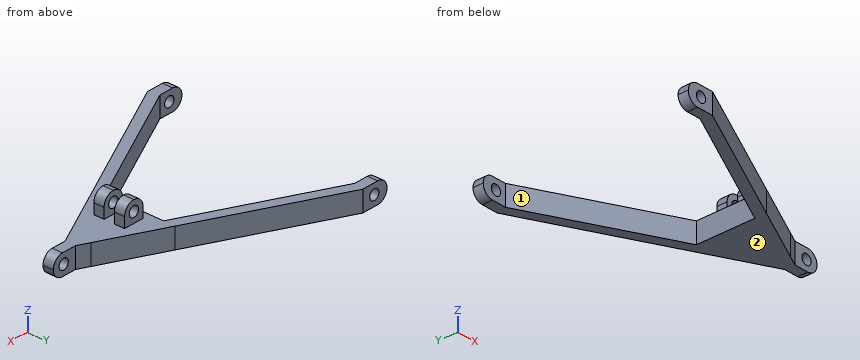
from build123d import *

# Parameters (mm, degrees)
EXTRUDE_THIN4_DEPTH = 20
SKETCH2_R           = 5
CUT_EXTRUDE1_DEPTH  = 235
BOSS_EXTRUDE1_DEPTH = 20
SKETCH4_W           = 20
SKETCH4_H           = 10
BOSS_EXTRUDE2_DEPTH = 20
SKETCH5_R           = 5
CUT_EXTRUDE2_DEPTH  = 160
FILLET1_R           = 10


# Read off the part's stored shape, not the designer's step: Extrude-Thin4
with BuildPart() as part:
    # Extrude-Thin4 outline → Extrude-Thin4 (new body)
    with BuildSketch(Plane.XY):
        Polygon((201.180339887, 5), (1.180339887, 105), (-25, 105), (-25, 95), (-1.180339887, 95), (188.819660113, 0), (-1.180339887, -95), (-25, -95), (-25, -105), (1.180339887, -105), (201.180339887, -5), (225, -5), (225, 5), align=None)
    extrude(amount=EXTRUDE_THIN4_DEPTH)

    # Sketch2 → Cut-Extrude1 (cut)
    with BuildSketch(Plane.XZ.offset(105)):
        with Locations(Location((-11.319660113, 10, 0), (0, 0, 270))):
            Circle(SKETCH2_R)
        with Locations(Location((213.680339887, 10, 0), (0, 0, 180))):
            Circle(SKETCH2_R)
    extrude(amount=-CUT_EXTRUDE1_DEPTH, mode=Mode.SUBTRACT)

    # Sketch3 → Boss-Extrude1 (add)
    with BuildSketch(Plane.XY.offset(20)):
        Polygon((131.729669907, -39.72533499), (131.729669907, 39.72533499), (190.16352069, 10.508409599), (190.16352069, -10.508409599), align=None)
    extrude(amount=-BOSS_EXTRUDE1_DEPTH)

    # Sketch4 → Boss-Extrude2 (add)
    with BuildSketch(Plane.XY.offset(20)):
        with Locations((148.953623882, -10)):
            Rectangle(SKETCH4_W, SKETCH4_H)
        with Locations((148.953623882, 10)):
            Rectangle(SKETCH4_W, SKETCH4_H)
    extrude(amount=BOSS_EXTRUDE2_DEPTH)

    # Sketch5 → Cut-Extrude2 (cut)
    with BuildSketch(Plane.XZ.offset(15)):
        with Locations(Location((148.953623882, 30, 0), (0, 0, 270))):
            Circle(SKETCH5_R)
    extrude(amount=-CUT_EXTRUDE2_DEPTH, mode=Mode.SUBTRACT)

    # Fillet1
    fillet1_edges = [part.edges().sort_by_distance(p)[0] for p in [
        (225, 0, 0),
        (225, 0, 20),
        (-25, 100, 0),
        (-25, 100, 20),
        (-25, -100, 0),
        (-25, -100, 20),
        (138.953623882, 10, 40),
        (158.953623882, 10, 40),
        (158.953623882, -10, 40),
        (138.953623882, -10, 40),
    ]]
    fillet(fillet1_edges, radius=FILLET1_R - 0.0001)  # a hair under: the kernel refuses the full size


solid = part.part
Model file for the job. Use its own axes, mm. Face numbers are marked on the shaded views. Coordinates: 2 decimals unless noted, no trailing zeros. Order: outer loops, then holes, each group sorted by start corner. A loop starts at its lowest first (then second) coordinate and runs counter-clockwise, first axis right, second up. Notation, with made-up numbers: (2.5, -8.75) -> (41.5, -8.75) arc R21 ccw to (41.5, 9.25) -> close; hole circle Ø10 at (2, 1). An arc over 180 degrees is marked (long way). Return JSON: item names as keys, results as strings. Group by question number.
Item 1: Pull direction Y, two halves, no side cores. Call the marked faces 1 and 2: pulls with the +Y half, pulls with the -Y half, needs draft (parallel to the pull), parting line crosses it, or undercut.
Item 2: Wall check: line 1 along X through (y, z) = (-8, 30); line 2 along X through (y, z) = (0, 10); line 3 along Y through (x, z) = (32.5, 6.5). Give the ranges that are in metal, low to high. Write a range as [from, to].
Item 3: Saw through at A-A on x = 71. Write the cut outline in (y, z).
Item 4: Flat gauge pins, fed straight in: P1, Ø1.5, axis at x = 129, z = 12, coming from the +Y side; P2, Ø6, axis at x = 150, z = 26.5, coming from the -Y side; P3, Ø11.5, axis at x = 213.68, z = 10, coming from the -Y side; P4, Ø11.5, axis at x = -11.32, z = 10, coming from the -Y side. Where does each tip first touch, or does it go through?
Values found:
{
 "1": {"face 1": "undercut", "face 2": "needs draft"},
 "2": {"line 1": "x = [138.95, 143.95], [153.95, 158.95]", "line 2": "x = [131.73, 208.68], [218.68, 225]", "line 3": "y = [-89.34, -78.16], [78.16, 89.34]"},
 "3": {"outline": "(-70.09, 0) -> (-58.91, 0) -> (-58.91, 20) -> (-70.09, 20) -> close; (58.91, 0) -> (70.09, 0) -> (70.09, 20) -> (58.91, 20) -> close"},
 "4": {"P1": "stops at y = 41.47", "P2": "stops at y = -15", "P3": "stops at y = -5", "P4": "stops at y = -105"}
}
